Build history of the part. All positions in model axes, mm. A direction names the side the tool comes from. Give positions to 0.01 mm unless a question says otherwise; leave off trailing zeros. Order: outer loops, then holes, each group sorted by start corner. A loop starts at its lowest first (then second) coordinate and runs counter-clockwise, first axis right, second up. Notation, with made-up numbers: M 65.25,32.5 L 106.25,32.5 A26 cw 106.25,58.5 Z; hole C 44,9.5 d5. An arc over 180 degrees is marked long. One line per item, written item: value.
from build123d import *

# Parameters (mm, degrees)
SKETCH1_R           = 5
BOSS_EXTRUDE1_DEPTH = 45
SKETCH2_R           = 3
BOSS_EXTRUDE2_DEPTH = 3
BOSS_EXTRUDE2_TAPER = 10
FILLET1_R           = 0.5


with BuildPart() as part:
    # Sketch1 → Boss-Extrude1 (new body)
    with BuildSketch(Plane(origin=(0, 0, 0), x_dir=(0, 0, -1), z_dir=(1, 0, 0))):
        Circle(SKETCH1_R)
    extrude(amount=BOSS_EXTRUDE1_DEPTH)

    # Sketch2 → Boss-Extrude2 (add)
    with BuildSketch(Plane.ZY):
        Circle(SKETCH2_R)
    extrude(amount=BOSS_EXTRUDE2_DEPTH, taper=BOSS_EXTRUDE2_TAPER)

    # Fillet1
    fillet1_edges = [part.edges().sort_by_distance(p)[0] for p in [
        (0, 0, 5),
        (-3, 0, -2.471019058),
    ]]
    fillet(fillet1_edges, radius=FILLET1_R)


solid = part.part
1) Tool access for faces 1 (the face through (0, -3, -1)), 2 (the face through (22.44, -4.88, 1.08)): list every direction of +Z, -Z, +X, -X, +Y, -Y with a clear straight run to the whole face (end or side of a thin tool).
Check values:
face 1: -X
face 2: +X, -X
2) Pin check, flat tips, straight feed: pin 1 (1.5 mm diameter, centred on x = 12, z = 3.5, fed in from +Y); pin 2 (3 mm diameter, centred on x = 38, y = -2, fed in from +Z). Stop position of each tip, or through.
Check values:
pin 1: y = 4.18
pin 2: z = 4.97
3) Saw through at B-B, the plane x = 32.5. Write the cut outline in (y, z), then the cut area to 3 significant figures.
Check values:
outline: C 0,0 d10
area: 78.5 mm^2
4) Drill centre lines: probe 1 along X at (y, z) = (2, 3.75); probe 2 along Z at (x, y) = (21, 4). Where is each one in solid material? Low to high. Write a range as from..to.
Check values:
probe 1: 0..45
probe 2: -3..3
5) Saw through at A-A, the plane z = 0. Write the cut outline in (x, y).
Check values:
outline: M -3,-2.05 A0.5 ccw -2.59,-2.54 L 0,-3 L 0,-4.5 A0.5 ccw 0.5,-5 L 45,-5 L 45,5 L 0.5,5 A0.5 ccw 0,4.5 L 0,3 L -2.59,2.54 A0.5 ccw -3,2.05 Z
